The listing builds one solid part. Answer for the finished solid, in the listing's coordinates (mm). A direction names the side the tool comes from. Round coordinates to 2 decimals unless told otherwise and drop trailing zeros. Answer as a JSON object with one key per item and string values.
```python
from build123d import *

# Parameters (mm, degrees)
F0_W      = 279.4
F0_H      = 330.2
F1_DEPTH  = 5.842
F2_W      = 25.4
F2_H      = 5.842
F2_W_2    = 76.2
F2_W_3    = 5.842
F2_H_2    = 25.4
F2_H_3    = 38.1
F3_DEPTH  = 5.842
F5_W      = 5.842
F5_H      = 12.7
F6_DEPTH  = 5.842
F7_DEPTH  = 5.842
F8_W      = 5.842
F8_H      = 25.4
F8_H_2    = 48.641
F8_H_3    = 34.925
F8_H_4    = 11.684
F9_DEPTH  = 5.842
F10_W     = 246.7240431406
F10_H     = 1.016
F11_DEPTH = 5.842
F13_W     = 25.4
F13_H     = 5.842
F13_W_2   = 19.558
F14_DEPTH = 5.842


# Not quite as in the source:
# - a feature names something its author has since deleted; it is built from what else it names


with BuildPart() as f1:
    # F0 (on Front) → F1 (new body)
    with BuildSketch(Plane.XZ):
        with Locations((25.751306051, 40.8756073241)):
            Rectangle(F0_W, F0_H)
    extrude(amount=F1_DEPTH)

    # F2 (on face) → F3 (cut, through all)
    with BuildSketch(Plane.XZ.offset(5.842)):
        with Locations((152.751306051, -121.3033926759)):
            Rectangle(F2_W, F2_H)
        with Locations((101.951306051, -121.3033926759)):
            Rectangle(F2_W, F2_H)
        with Locations((51.151306051, -121.3033926759)):
            Rectangle(F2_W, F2_H)
        with Locations((0.351306051, -121.3033926759)):
            Rectangle(F2_W, F2_H)
        with Locations((-75.848693949, -121.3033926759)):
            Rectangle(F2_W_2, F2_H)
        with Locations((162.530306051, -86.1243926759)):
            Rectangle(F2_W_3, F2_H_2)
        with Locations((162.530306051, -28.9743926759)):
            Rectangle(F2_W_3, F2_H_3)
        with Locations((-111.027693949, -86.1243926759)):
            Rectangle(F2_W_3, F2_H_2)
        with Locations((-111.027693949, -35.3243926759)):
            Rectangle(F2_W_3, F2_H_2)
        with Locations((-111.027693949, 15.4756073241)):
            Rectangle(F2_W_3, F2_H_2)
        with Locations((-111.027693949, 66.2756073241)):
            Rectangle(F2_W_3, F2_H_2)
        with Locations((-111.027693949, 167.8756073241)):
            Rectangle(F2_W_3, F2_H_2)
        with Locations((-111.027693949, 117.0756073241)):
            Rectangle(F2_W_3, F2_H_2)
    extrude(amount=-F3_DEPTH, mode=Mode.SUBTRACT)

    # F5 (on face) → F6 (cut, through all)
    with BuildSketch(Plane.XZ.offset(5.842)):
        with Locations((162.530306051, 2.7756073241)):
            Rectangle(F5_W, F5_H)
    extrude(amount=-F6_DEPTH, mode=Mode.SUBTRACT)

    # F4 (on face) → F7 (cut, through all)
    with BuildSketch(Plane.XZ.offset(5.842)):
        with BuildLine():
            Line((165.451306051, 15.4756073241), (159.609306051, 15.4756073241))
            add(Edge.make_bspline(
                [(159.609306051, 15.4756073241), (73.376306051, 28.1756073241), (-24.3765935073, 60.3637718481), (-21.873693949, 193.2756073241), (-113.948693949, 205.9756073241)],
                knots=[0, 0, 0, 0, 0.507272, 1, 1, 1, 1], degree=3))
            Line((-113.948693949, 205.9756073241), (-113.948693949, 180.5756073241))
            Line((-113.948693949, 180.5756073241), (-108.106693949, 180.5756073241))
            Line((-108.106693949, 180.5756073241), (-108.106693949, 155.1756073241))
            Line((-108.106693949, 155.1756073241), (-113.948693949, 155.1756073241))
            Line((-113.948693949, 155.1756073241), (-113.948693949, 129.7756073241))
            Line((-113.948693949, 129.7756073241), (-108.106693949, 129.7756073241))
            Line((-108.106693949, 129.7756073241), (-108.106693949, 104.3756073241))
            Line((-108.106693949, 104.3756073241), (-113.948693949, 104.3756073241))
            Line((-113.948693949, 104.3756073241), (-113.948693949, 78.9756073241))
            Line((-113.948693949, 78.9756073241), (-108.106693949, 78.9756073241))
            Line((-108.106693949, 78.9756073241), (-108.106693949, 53.5756073241))
            Line((-108.106693949, 53.5756073241), (-113.948693949, 53.5756073241))
            Line((-113.948693949, 53.5756073241), (-113.948693949, 28.1756073241))
            Line((-113.948693949, 28.1756073241), (-108.106693949, 28.1756073241))
            Line((-108.106693949, 28.1756073241), (-108.106693949, 2.7756073241))
            Line((-108.106693949, 2.7756073241), (-113.948693949, 2.7756073241))
            Line((-113.948693949, 2.7756073241), (-113.948693949, -22.6243926759))
            Line((-113.948693949, -22.6243926759), (-108.106693949, -22.6243926759))
            Line((-108.106693949, -22.6243926759), (-108.106693949, -48.0243926759))
            Line((-108.106693949, -48.0243926759), (-113.948693949, -48.0243926759))
            Line((-113.948693949, -48.0243926759), (-113.948693949, -73.4243926759))
            Line((-113.948693949, -73.4243926759), (-108.106693949, -73.4243926759))
            Line((-108.106693949, -73.4243926759), (-108.106693949, -98.8243926759))
            Line((-108.106693949, -98.8243926759), (-113.948693949, -98.8243926759))
            Line((-113.948693949, -98.8243926759), (-113.948693949, -118.3823926759))
            Line((-113.948693949, -118.3823926759), (-37.748693949, -118.3823926759))
            Line((-37.748693949, -118.3823926759), (-37.748693949, -124.2243926759))
            Line((-37.748693949, -124.2243926759), (-12.348693949, -124.2243926759))
            Line((-12.348693949, -124.2243926759), (-12.348693949, -118.3823926759))
            Line((-12.348693949, -118.3823926759), (13.051306051, -118.3823926759))
            Line((13.051306051, -118.3823926759), (13.051306051, -124.2243926759))
            Line((13.051306051, -124.2243926759), (38.451306051, -124.2243926759))
            Line((38.451306051, -124.2243926759), (38.451306051, -118.3823926759))
            Line((38.451306051, -118.3823926759), (63.851306051, -118.3823926759))
            Line((63.851306051, -118.3823926759), (63.851306051, -124.2243926759))
            Line((63.851306051, -124.2243926759), (89.251306051, -124.2243926759))
            Line((89.251306051, -124.2243926759), (89.251306051, -118.3823926759))
            Line((89.251306051, -118.3823926759), (114.651306051, -118.3823926759))
            Line((114.651306051, -118.3823926759), (114.651306051, -124.2243926759))
            Line((114.651306051, -124.2243926759), (140.051306051, -124.2243926759))
            Line((140.051306051, -124.2243926759), (140.051306051, -118.3823926759))
            Line((140.051306051, -118.3823926759), (165.451306051, -118.3823926759))
            Line((165.451306051, -118.3823926759), (165.451306051, -98.8243926759))
            Line((165.451306051, -98.8243926759), (159.609306051, -98.8243926759))
            Line((159.609306051, -98.8243926759), (159.609306051, -73.4243926759))
            Line((159.609306051, -73.4243926759), (165.451306051, -73.4243926759))
            Line((165.451306051, -73.4243926759), (165.451306051, -48.0243926759))
            Line((165.451306051, -48.0243926759), (159.609306051, -48.0243926759))
            Line((159.609306051, -48.0243926759), (159.609306051, -9.9243926759))
            Line((159.609306051, -9.9243926759), (165.451306051, -9.9243926759))
            Line((165.451306051, -9.9243926759), (165.451306051, 15.4756073241))
        make_face()
        with BuildLine():
            add(Edge.make_bspline(
                [(159.609306051, 15.4756073241), (73.376306051, 28.1756073241), (-24.3765935073, 60.3637718481), (-21.873693949, 193.2756073241), (-113.948693949, 205.9756073241)],
                knots=[0, 0, 0, 0, 0.507272, 1, 1, 1, 1], degree=3))
            Line((159.609306051, 15.4756073241), (159.609306051, 21.8256073241))
            add(Edge.make_bspline(
                [(159.609306051, 21.8256073241), (63.851306051, 34.5256073241), (-5.6173037023, 95.4914607938), (-31.4644745687, 187.7697107475), (-87.114737086, 205.9756073241)],
                knots=[0, 0, 0, 0, 0.5236819738, 0.940243193, 0.940243193, 0.940243193, 0.940243193], degree=3))
            Line((-87.114737086, 205.9756073241), (-113.948693949, 205.9756073241))
        make_face()
    extrude(amount=-F7_DEPTH, mode=Mode.SUBTRACT)

    # F8 (on face) → F9 (cut, through all)
    with BuildSketch(Plane.XZ.offset(5.842)):
        Polygon((165.451306051, 15.4756073241), (165.451306051, 28.1756073241), (159.609306051, 28.1756073241), (159.609306051, 21.8256073241), (159.609306051, 15.4756073241), align=None)
        with Locations((162.530306051, 40.8756073241)):
            Rectangle(F8_W, F8_H)
        with Locations((162.530306051, 77.8961073241)):
            Rectangle(F8_W, F8_H_2)
        with BuildLine():
            Line((159.609306051, 102.2166073241), (165.451306051, 102.2166073241))
            Line((165.451306051, 102.2166073241), (165.451306051, 103.3306229057))
            ThreePointArc((165.451306051, 103.3306229057), (162.5829399691, 102.4975980153), (159.609306051, 102.2166073241))
        make_face()
        with BuildLine():
            ThreePointArc((145.861152343, 110.1541080567), (151.6718056847, 104.3434542505), (159.609306051, 102.2166073241))
            Line((159.609306051, 102.2166073241), (159.609306051, 133.9666073241))
            ThreePointArc((159.609306051, 133.9666073241), (151.6718056847, 131.8397603977), (145.861152343, 126.0291065915))
            ThreePointArc((145.861152343, 126.0291065915), (143.734306051, 118.0916073241), (145.861152343, 110.1541080567))
        make_face()
        with BuildLine():
            Line((150.4438705276, 102.2166073241), (159.609306051, 102.2166073241))
            ThreePointArc((159.609306051, 102.2166073241), (151.6718056847, 104.3434542505), (145.861152343, 110.1541080567))
            Line((145.861152343, 110.1541080567), (150.4438705276, 102.2166073241))
        make_face()
        with BuildLine():
            Line((159.609306051, 133.9666073241), (159.609306051, 102.2166073241))
            ThreePointArc((159.609306051, 102.2166073241), (162.5829399691, 102.4975980153), (165.451306051, 103.3306229057))
            Line((165.451306051, 103.3306229057), (165.451306051, 132.8525917425))
            ThreePointArc((165.451306051, 132.8525917425), (162.5829399691, 133.6856166328), (159.609306051, 133.9666073241))
        make_face()
        with BuildLine():
            Line((165.451306051, 133.9666073241), (159.609306051, 133.9666073241))
            ThreePointArc((159.609306051, 133.9666073241), (162.5829399691, 133.6856166328), (165.451306051, 132.8525917425))
            Line((165.451306051, 132.8525917425), (165.451306051, 133.9666073241))
        make_face()
        with BuildLine():
            ThreePointArc((145.861152343, 126.0291065915), (151.6718056847, 131.8397603977), (159.609306051, 133.9666073241))
            Line((159.609306051, 133.9666073241), (150.4438705276, 133.9666073241))
            Line((150.4438705276, 133.9666073241), (145.861152343, 126.0291065915))
        make_face()
        with Locations((162.530306051, 151.4291073241)):
            Rectangle(F8_W, F8_H_3)
        with BuildLine():
            Line((141.2784350042, 118.0916073241), (145.861152343, 110.1541080567))
            ThreePointArc((145.861152343, 110.1541080567), (143.734306051, 118.0916073241), (145.861152343, 126.0291065915))
            Line((145.861152343, 126.0291065915), (141.2784350042, 118.0916073241))
        make_face()
        with Locations((162.530306051, 200.1336073241)):
            Rectangle(F8_W, F8_H_4)
    extrude(amount=-F9_DEPTH, mode=Mode.SUBTRACT)

    # F10 (on face) → F11 (join, through all)
    with BuildSketch(Plane.XZ.offset(5.842)):
        with Locations((36.2472844807, 206.4836073241)):
            Rectangle(F10_W, F10_H)
    extrude(amount=-F11_DEPTH)

    # F13 (on face) → F14 (cut, through all)
    with BuildSketch(Plane.XZ.offset(5.842)):
        with Locations((51.151306051, 204.0706073241)):
            Rectangle(F13_W, F13_H)
        with Locations((101.951306051, 204.0706073241)):
            Rectangle(F13_W, F13_H)
        with Locations((149.830306051, 204.0706073241)):
            Rectangle(F13_W_2, F13_H)
        with BuildLine():
            add(Edge.make_bspline(
                [(-64.0656111495, 195.8912068503), (-64.4986133811, 197.8821506555), (-64.5462177809, 200.9608220943), (-64.8897370896, 206.9916073241)],
                knots=[0.7783755915, 0.7783755915, 0.7783755915, 0.7783755915, 1, 1, 1, 1], degree=3))
            Line((-64.8897370896, 206.9916073241), (-87.1147370896, 206.9916073241))
            Line((-87.1147370896, 206.9916073241), (-87.1147370896, 205.9756073241))
            add(Edge.make_bspline(
                [(-64.0656111419, 195.8912068549), (-70.8038372609, 199.7329606353), (-78.4197996839, 203.1310721158), (-87.114737086, 205.9756073241)],
                knots=[0.8751586172, 0.8751586172, 0.8751586172, 0.8751586172, 0.940243193, 0.940243193, 0.940243193, 0.940243193], degree=3))
        make_face()
        with Locations((0.351306051, 204.0706073241)):
            Rectangle(F13_W, F13_H)
        with BuildLine():
            Line((-63.148693949, 195.362557311), (-63.148693949, 206.9916073241))
            Line((-63.148693949, 206.9916073241), (-64.8897370896, 206.9916073241))
            add(Edge.make_bspline(
                [(-64.0656111495, 195.8912068503), (-64.4986133811, 197.8821506555), (-64.5462177809, 200.9608220943), (-64.8897370896, 206.9916073241)],
                knots=[0.7783755915, 0.7783755915, 0.7783755915, 0.7783755915, 1, 1, 1, 1], degree=3))
            add(Edge.make_bspline(
                [(-63.148693949, 195.362557311), (-63.4525182871, 195.5396905387), (-63.7581509788, 195.7159105346), (-64.0656111419, 195.8912068549)],
                knots=[0.8721888572, 0.8721888572, 0.8721888572, 0.8721888572, 0.8751586172, 0.8751586172, 0.8751586172, 0.8751586172], degree=3))
        make_face()
    extrude(amount=-F14_DEPTH, mode=Mode.SUBTRACT)


solid = f1.part
```
Item 1: Flat-ended cylindrical pins translate along their axes: P1, Ø1.8, axis at y = -3.5, z = 205, coming from the +X side; P2, Ø1, axis at y = -3.5, z = 106, coming from the +X side; P3, Ø1.8, axis at x = 155.5, y = -2, coming from the +Z side. Find the tip coordinate at first contact, or state that the pin passes through.
Values follow:
{"P1": "x = 140.05", "P2": "x = 148.55", "P3": "z = 201.15"}
Item 2: Determine the mould class of faces 1 (the face through (155, -3, 102.217)), 2 (the face through (150, -3, 201.15)), 3 (the face through (159.609, -3, 198)) for opening direction Z: released by +Z, released by -Z, zero draft, split by the parting line, or undercut.
Values follow:
{"face 1": "undercut", "face 2": "released by +Z", "face 3": "zero draft"}
Item 3: Straight lines are drawn through the part: line 1 (X direction, y = -5.45, z = 157); line 2 (Z direction, x = 45, y = -1.25); line 3 (X direction, y = -4.75, z = 62). For each, find the intervals that lie inside material, in ascending order.
Values follow:
{"line 1": "-24.57 to 159.61", "line 2": "60.97 to 201.15", "line 3": "43.59 to 159.61"}
Item 4: Which of the six approach directions +Z, -Z, +X, -X, +Y, -Y give full straight-line access (tool end or side, diameter ignored) to faces 4 (the face through (165.451, -3, 181)), 5 (the face through (-63.149, -3, 201)), 6 (the face through (159.609, -3, 151)), 7 (the face through (140.051, -3, 204)), 8 (the face through (89.251, -3, 204))?
Values follow:
{"face 4": "+Z, -Z, +X, +Y, -Y", "face 5": "+Z, -Z, -X, +Y, -Y", "face 6": "-Z, +X, +Y, -Y", "face 7": "+Z, +X, +Y, -Y", "face 8": "+Z, +Y, -Y"}
